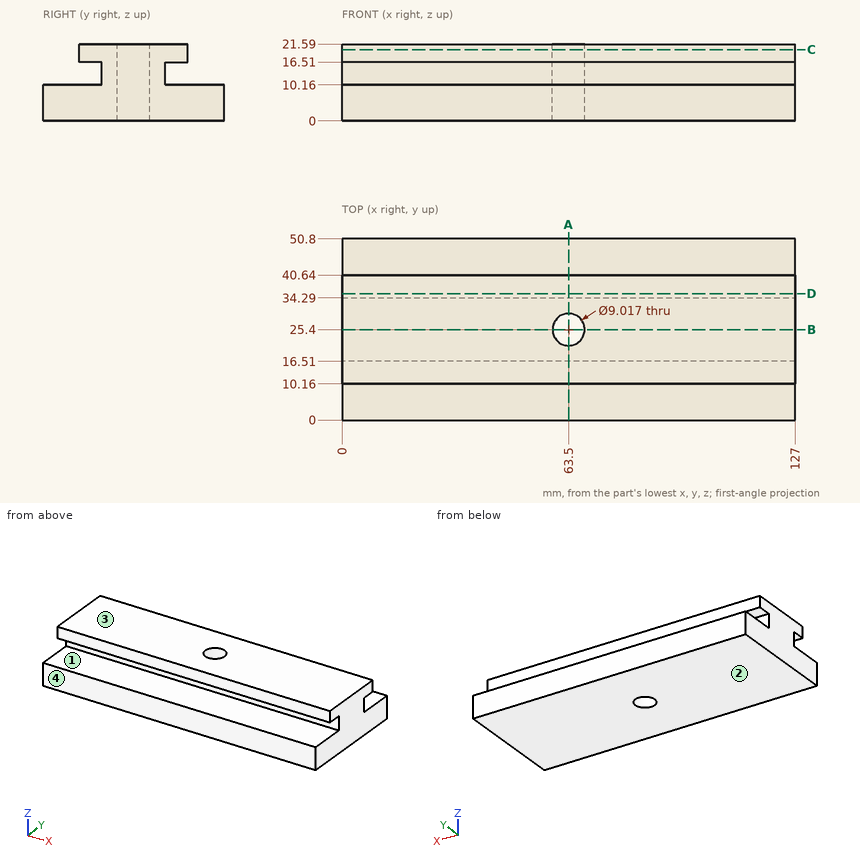
Here's the drawing with two shaded views (mm, measured from the low corner). I have some questions. Round coordinates to 2 decimals unless told otherwise and drop trailing zeros. Write each loop counter-clockwise with the first axis right and the second up, starting at its lowest first coordinate (ties: lowest second). Pieces come first, ordered by that corner, then holes. Notation, with made-up numbers: M 39.5,-26.5 L 58.5,-26.5 A30 ccw 58.5,-2.5 Z; hole C 85,-15 d6. An arc over 180 degrees is marked long. Use CSV: the item, a comma, the result in double quotes.
(1) I need wall thicknesses on line 1 along Y through (x, z) = (63.5, 9.5); line 2 along Z through (x, y) = (41, 36); line 3 along X through (y, z) = (25.4, 9.75). Which ranges of each line are inside material? Lowest first, please.
Check values:
line 1,"0 to 20.89, 29.91 to 50.8"
line 2,"0 to 10.16, 16.51 to 21.59"
line 3,"0 to 58.99, 68.01 to 127"
(2) Imagine slicing it at D-D (y = 35.5). Write out the boundary of the cut face in (x, z).
Check values:
outline,"M 0,0 L 127,0 L 127,10.16 L 0,10.16 Z; M 0,16.51 L 127,16.51 L 127,21.59 L 0,21.59 Z"
(3) Imagine slicing it at C-C (z = 20). Write out the boundary of the cut face in (x, y), plus the area to 3 significant figures.
Check values:
outline,"M 0,10.16 L 127,10.16 L 127,40.64 L 0,40.64 Z; hole C 63.5,25.4 d9.02"
area,"3,810 mm^2"
(4) I'm going to push flat-ended pins straight in: pin 1 (3 mm diameter, centred on x = 44.5, z = 12.5, fed in from +Y); pin 2 (5.5 mm diameter, centred on x = 92.5, z = 19, fed in from +Y); pin 3 (1.9 mm diameter, centred on x = 77, z = 13.5, fed in from -Y). Where does each tip first touch, or does it pass through?
Check values:
pin 1,"y = 34.29"
pin 2,"y = 40.64"
pin 3,"y = 16.51"
(5) We'd pull the mould along Z, two halves only. Please class the marked faces 1, 2, 3 and 4: +Z half, -Z half, draft (parallel to the pull), parting line (faces both ways), or undercut.
Check values:
face 1,"undercut"
face 2,"-Z half"
face 3,"+Z half"
face 4,"draft"
(6) Imagine slicing it at B-B (y = 25.4). Write out the boundary of the cut face in (x, z).
Check values:
outline,"M 0,0 L 58.99,0 L 58.99,21.59 L 0,21.59 Z; M 68.01,0 L 127,0 L 127,21.59 L 68.01,21.59 Z"
(7) Imagine slicing it at A-A (x = 63.5). Write out the boundary of the cut face in (y, z), plus the area to 3 significant figures.
Check values:
outline,"M 0,0 L 20.89,0 L 20.89,21.59 L 10.16,21.59 L 10.16,16.51 L 16.51,16.51 L 16.51,10.16 L 0,10.16 Z; M 29.91,0 L 50.8,0 L 50.8,10.16 L 34.29,10.16 L 34.29,16.51 L 40.64,16.51 L 40.64,21.59 L 29.91,21.59 Z"
area,"589 mm^2"
